Check sheet for the drawn part. Datum: minimum x, y, z corner. Units: mm. Round coordinates to 2 decimals unless told otherwise and drop trailing zeros. Write each loop counter-clockwise with the first axis right and the second up, starting at its lowest first coordinate (ties: lowest second). Pieces come first, ordered by that corner, then holes. Notation, with made-up numbers: (31, 5.25) -> (35, 5.25) arc R22 cw to (35, 39.25) -> close; hole circle Ø9 at (12.25, 1). An arc over 180 degrees is marked (long way). Use CSV: the item, a comma, the result in double quotes.
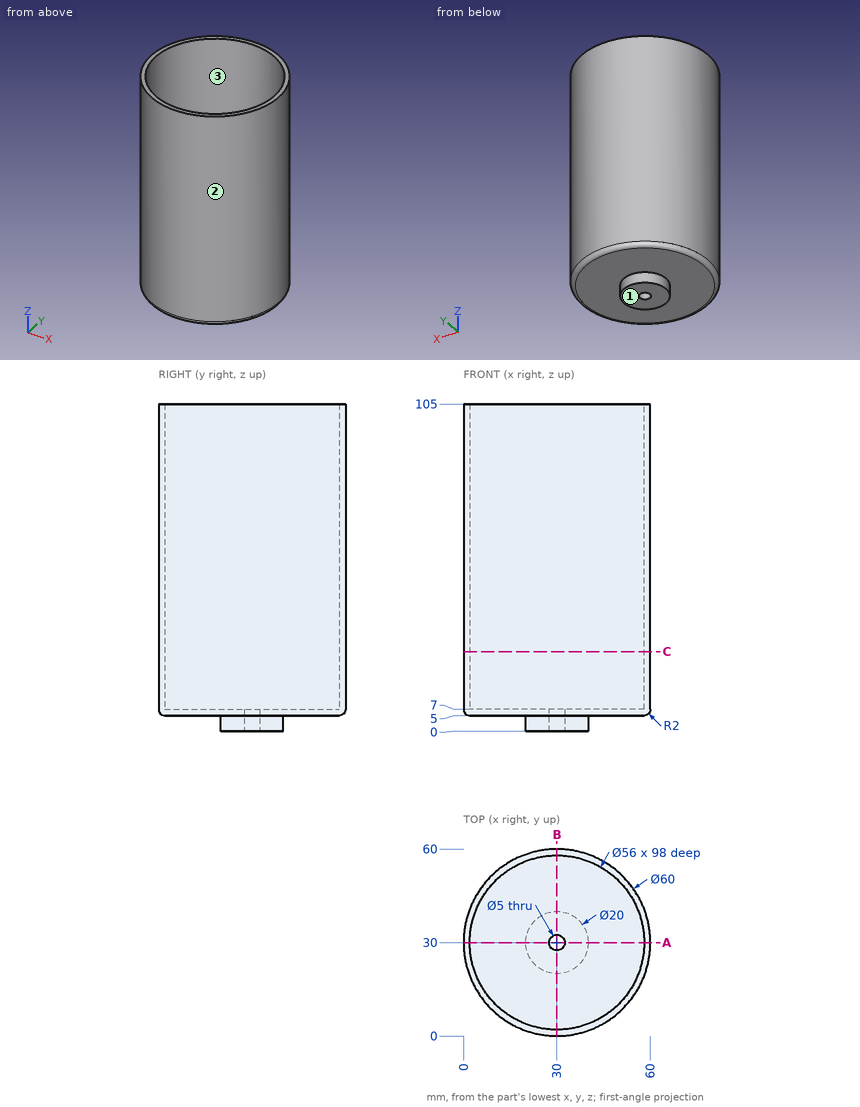
Q1. Go/stop test with flat-tipped pins: P1, Ø5, axis at x = 38, y = 9.5, coming from the +Z side; P2, Ø2, axis at x = 9, z = 51.5, coming from the -Y side; P3, Ø1, axis at x = 34, y = 21, coming from the -Z side; P4, Ø4, axis at x = 49, z = 72, coming from the +Y side. Record where each tip stops, or that it passes through.
Filled in:
P1,"z = 7"
P2,"y = 7.64"
P3,"z = 0"
P4,"y = 54.72"
Q2. Section check A-A (y = 30). Record the cut outline in (x, z), plus the area to 3 significant figures.
Filled in:
outline,"(0, 7) arc R2 ccw to (2, 5) -> (20, 5) -> (20, 0) -> (27.5, 0) -> (27.5, 7) -> (2, 7) -> (2, 105) -> (0, 105) -> close; (32.5, 0) -> (40, 0) -> (40, 5) -> (58, 5) arc R2 ccw to (60, 7) -> (60, 105) -> (58, 105) -> (58, 7) -> (32.5, 7) -> close"
area,"575 mm²"
Q3. Section check C-C (z = 25.5). Record the cut outline in (x, y).
Filled in:
outline,"circle Ø60 at (30, 30); hole circle Ø56 at (30, 30)"
Q4. Material ranges on L1, parallel to Y at x = 30, z = 53; L2, parallel to Y at x = 30, z = 3.75; L3, parallel to Z at x = 8, y = 40.5, recorded low to high.
Filled in:
L1,"0 to 2, 58 to 60"
L2,"20 to 27.5, 32.5 to 40"
L3,"5 to 7"
Q5. Mould release check, pull along Y, two halves, no side actions. Record for the marked faces 1, 2 and 3: released by +Y, released by -Y, zero draft, split by the parting line, or undercut.
Filled in:
face 1,"zero draft"
face 2,"split by the parting line"
face 3,"undercut"
